from build123d import *

# Parameters (mm, degrees)
EXTRUDE_1_DEPTH = 100


with BuildPart() as part:
    # Model → 凸台-拉伸1 (new body)
    with BuildSketch(Plane.XY):
        with BuildLine():
            Line((1440.867570561, 579.107478259), (1452.807293918, 579.107478259))
            Line((1452.807293918, 579.107478259), (1457.807293918, 579.107478259))
            ThreePointArc((1457.807293918, 579.107478259), (1458.019425952, 579.019610294), (1458.107293918, 578.807478259))
            Line((1458.107293918, 578.807478259), (1458.107293918, 577.507478259))
            ThreePointArc((1458.107293918, 577.507478259), (1458.019425952, 577.295346225), (1457.807293918, 577.207478259))
            Line((1457.807293918, 577.207478259), (1408.407293918, 577.207478259))
            ThreePointArc((1408.407293918, 577.207478259), (1408.195161884, 577.295346225), (1408.107293918, 577.507478259))
            Line((1408.107293918, 577.507478259), (1408.107293918, 578.807478259))
            ThreePointArc((1408.107293918, 578.807478259), (1408.195161884, 579.019610294), (1408.407293918, 579.107478259))
            Line((1408.407293918, 579.107478259), (1425.347017276, 579.107478259))
            ThreePointArc((1425.347017276, 579.107478259), (1425.700570666, 579.253924869), (1425.847017276, 579.607478259))
            Line((1425.847017276, 579.607478259), (1425.847017276, 582.022074556))
            ThreePointArc((1425.847017276, 582.022074556), (1425.888989436, 582.222600109), (1426.007859266, 582.389459701))
            Line((1426.007859266, 582.389459701), (1427.136441813, 583.431330379))
            ThreePointArc((1427.136441813, 583.431330379), (1427.231524995, 583.680936543), (1427.089921929, 583.907415283))
            ThreePointArc((1427.089921929, 583.907415283), (1424.975565934, 585.575750276), (1423.307230942, 587.69010627))
            ThreePointArc((1423.307230942, 587.69010627), (1423.080752201, 587.831709337), (1422.831146038, 587.736626154))
            Line((1422.831146038, 587.736626154), (1421.789275359, 586.608043608))
            ThreePointArc((1421.789275359, 586.608043608), (1421.366754977, 586.450250809), (1420.989097485, 586.696821001))
            ThreePointArc((1420.989097485, 586.696821001), (1419.107293918, 593.707478259), (1420.989097485, 600.718135518))
            ThreePointArc((1420.989097485, 600.718135518), (1421.366754977, 600.96470571), (1421.789275359, 600.806912911))
            Line((1421.789275359, 600.806912911), (1422.831146038, 599.678330364))
            ThreePointArc((1422.831146038, 599.678330364), (1423.080752201, 599.583247182), (1423.307230942, 599.724850249))
            ThreePointArc((1423.307230942, 599.724850249), (1424.975565934, 601.839206243), (1427.089921929, 603.507541236))
            ThreePointArc((1427.089921929, 603.507541236), (1427.231524995, 603.734019976), (1427.136441813, 603.98362614))
            Line((1427.136441813, 603.98362614), (1426.007859266, 605.025496818))
            ThreePointArc((1426.007859266, 605.025496818), (1425.850066468, 605.448017201), (1426.096636659, 605.825674693))
            ThreePointArc((1426.096636659, 605.825674693), (1433.107293918, 607.707478259), (1440.117951177, 605.825674693))
            ThreePointArc((1440.117951177, 605.825674693), (1440.364521369, 605.448017201), (1440.20672857, 605.025496818))
            Line((1440.20672857, 605.025496818), (1439.078146023, 603.98362614))
            ThreePointArc((1439.078146023, 603.98362614), (1438.983062841, 603.734019976), (1439.124665907, 603.507541236))
            ThreePointArc((1439.124665907, 603.507541236), (1441.239021902, 601.839206243), (1442.907356895, 599.724850249))
            ThreePointArc((1442.907356895, 599.724850249), (1443.133835635, 599.583247182), (1443.383441798, 599.678330364))
            Line((1443.383441798, 599.678330364), (1444.425312477, 600.806912911))
            ThreePointArc((1444.425312477, 600.806912911), (1444.847832859, 600.96470571), (1445.225490352, 600.718135518))
            ThreePointArc((1445.225490352, 600.718135518), (1447.107293918, 593.707478259), (1445.225490352, 586.696821001))
            ThreePointArc((1445.225490352, 586.696821001), (1444.847832859, 586.450250809), (1444.425312477, 586.608043608))
            Line((1444.425312477, 586.608043608), (1443.383441798, 587.736626154))
            ThreePointArc((1443.383441798, 587.736626154), (1443.133835635, 587.831709337), (1442.907356895, 587.69010627))
            ThreePointArc((1442.907356895, 587.69010627), (1441.239021902, 585.575750276), (1439.124665907, 583.907415283))
            ThreePointArc((1439.124665907, 583.907415283), (1438.983062841, 583.680936543), (1439.078146023, 583.431330379))
            Line((1439.078146023, 583.431330379), (1440.20672857, 582.389459701))
            ThreePointArc((1440.20672857, 582.389459701), (1440.325598401, 582.222600109), (1440.367570561, 582.022074556))
            Line((1440.367570561, 582.022074556), (1440.367570561, 579.607478259))
            ThreePointArc((1440.367570561, 579.607478259), (1440.51401717, 579.253924869), (1440.867570561, 579.107478259))
        make_face()
        with BuildLine():
            Line((1421.166188442, 590.907478259), (1421.754066124, 590.907478259))
            ThreePointArc((1421.754066124, 590.907478259), (1421.914408846, 590.857021745), (1422.016963461, 590.723836915))
            Line((1422.016963461, 590.723836915), (1422.411999107, 589.64605289))
            ThreePointArc((1422.411999107, 589.64605289), (1422.514553722, 589.51286806), (1422.674896444, 589.462411545))
            Line((1422.674896444, 589.462411545), (1424.424991887, 589.462411545))
            ThreePointArc((1424.424991887, 589.462411545), (1424.58032957, 589.419063458), (1424.690776643, 589.30154624))
            ThreePointArc((1424.690776643, 589.30154624), (1426.389779497, 586.989963838), (1428.701361899, 585.290960984))
            ThreePointArc((1428.701361899, 585.290960984), (1428.818879117, 585.180513911), (1428.862227204, 585.025176228))
            Line((1428.862227204, 585.025176228), (1428.862227204, 583.275080785))
            ThreePointArc((1428.862227204, 583.275080785), (1428.912683718, 583.114738064), (1429.045868549, 583.012183448))
            Line((1429.045868549, 583.012183448), (1430.123652573, 582.617147802))
            ThreePointArc((1430.123652573, 582.617147802), (1430.256837404, 582.514593187), (1430.307293918, 582.354250466))
            Line((1430.307293918, 582.354250466), (1430.307293918, 581.766372783))
            ThreePointArc((1430.307293918, 581.766372783), (1430.374439218, 581.577220229), (1430.545818508, 581.472739042))
            ThreePointArc((1430.545818508, 581.472739042), (1433.107293918, 581.207478259), (1435.668769328, 581.472739042))
            ThreePointArc((1435.668769328, 581.472739042), (1435.840148618, 581.577220229), (1435.907293918, 581.766372783))
            Line((1435.907293918, 581.766372783), (1435.907293918, 582.354250466))
            ThreePointArc((1435.907293918, 582.354250466), (1435.957750433, 582.514593187), (1436.090935263, 582.617147802))
            Line((1436.090935263, 582.617147802), (1437.168719288, 583.012183448))
            ThreePointArc((1437.168719288, 583.012183448), (1437.301904118, 583.114738064), (1437.352360632, 583.275080785))
            Line((1437.352360632, 583.275080785), (1437.352360632, 585.025176228))
            ThreePointArc((1437.352360632, 585.025176228), (1437.39570872, 585.180513911), (1437.513225937, 585.290960984))
            ThreePointArc((1437.513225937, 585.290960984), (1439.824808339, 586.989963838), (1441.523811193, 589.30154624))
            ThreePointArc((1441.523811193, 589.30154624), (1441.634258267, 589.419063458), (1441.789595949, 589.462411545))
            Line((1441.789595949, 589.462411545), (1443.539691393, 589.462411545))
            ThreePointArc((1443.539691393, 589.462411545), (1443.700034114, 589.51286806), (1443.802588729, 589.64605289))
            Line((1443.802588729, 589.64605289), (1444.197624375, 590.723836915))
            ThreePointArc((1444.197624375, 590.723836915), (1444.300178991, 590.857021745), (1444.460521712, 590.907478259))
            Line((1444.460521712, 590.907478259), (1445.048399395, 590.907478259))
            ThreePointArc((1445.048399395, 590.907478259), (1445.237551948, 590.974623559), (1445.342033136, 591.14600285))
            ThreePointArc((1445.342033136, 591.14600285), (1445.607293918, 593.707478259), (1445.342033136, 596.268953669))
            ThreePointArc((1445.342033136, 596.268953669), (1445.237551948, 596.44033296), (1445.048399395, 596.507478259))
            Line((1445.048399395, 596.507478259), (1444.460521712, 596.507478259))
            ThreePointArc((1444.460521712, 596.507478259), (1444.300178991, 596.557934774), (1444.197624375, 596.691119604))
            Line((1444.197624375, 596.691119604), (1443.802588729, 597.768903629))
            ThreePointArc((1443.802588729, 597.768903629), (1443.700034114, 597.902088459), (1443.539691393, 597.952544974))
            Line((1443.539691393, 597.952544974), (1441.789595949, 597.952544974))
            ThreePointArc((1441.789595949, 597.952544974), (1441.634258267, 597.995893061), (1441.523811193, 598.113410278))
            ThreePointArc((1441.523811193, 598.113410278), (1440.851379085, 599.210127161), (1440.036940374, 600.205939616))
            Line((1440.036940374, 600.205939616), (1440.036940374, 600.637124715))
            Line((1440.036940374, 600.637124715), (1439.605755274, 600.637124715))
            ThreePointArc((1439.605755274, 600.637124715), (1438.609942819, 601.451563426), (1437.513225937, 602.123995535))
            ThreePointArc((1437.513225937, 602.123995535), (1437.39570872, 602.234442608), (1437.352360632, 602.389780291))
            Line((1437.352360632, 602.389780291), (1437.352360632, 604.139875734))
            ThreePointArc((1437.352360632, 604.139875734), (1437.301904118, 604.300218455), (1437.168719288, 604.402773071))
            Line((1437.168719288, 604.402773071), (1436.090935263, 604.797808717))
            ThreePointArc((1436.090935263, 604.797808717), (1435.957750433, 604.900363332), (1435.907293918, 605.060706053))
            Line((1435.907293918, 605.060706053), (1435.907293918, 605.648583736))
            ThreePointArc((1435.907293918, 605.648583736), (1435.840148618, 605.837736289), (1435.668769328, 605.942217477))
            ThreePointArc((1435.668769328, 605.942217477), (1433.107293918, 606.207478259), (1430.545818508, 605.942217477))
            ThreePointArc((1430.545818508, 605.942217477), (1430.374439218, 605.837736289), (1430.307293918, 605.648583736))
            Line((1430.307293918, 605.648583736), (1430.307293918, 605.060706053))
            ThreePointArc((1430.307293918, 605.060706053), (1430.256837404, 604.900363332), (1430.123652573, 604.797808717))
            Line((1430.123652573, 604.797808717), (1429.045868549, 604.402773071))
            ThreePointArc((1429.045868549, 604.402773071), (1428.912683718, 604.300218455), (1428.862227204, 604.139875734))
            Line((1428.862227204, 604.139875734), (1428.862227204, 602.389780291))
            ThreePointArc((1428.862227204, 602.389780291), (1428.818879117, 602.234442608), (1428.701361899, 602.123995535))
            ThreePointArc((1428.701361899, 602.123995535), (1426.389779497, 600.424992681), (1424.690776643, 598.113410278))
            ThreePointArc((1424.690776643, 598.113410278), (1424.58032957, 597.995893061), (1424.424991887, 597.952544974))
            Line((1424.424991887, 597.952544974), (1422.674896444, 597.952544974))
            ThreePointArc((1422.674896444, 597.952544974), (1422.514553722, 597.902088459), (1422.411999107, 597.768903629))
            Line((1422.411999107, 597.768903629), (1422.016963461, 596.691119604))
            ThreePointArc((1422.016963461, 596.691119604), (1421.914408846, 596.557934774), (1421.754066124, 596.507478259))
            Line((1421.754066124, 596.507478259), (1421.166188442, 596.507478259))
            ThreePointArc((1421.166188442, 596.507478259), (1420.977035888, 596.44033296), (1420.8725547, 596.268953669))
            ThreePointArc((1420.8725547, 596.268953669), (1420.607293918, 593.707478259), (1420.8725547, 591.14600285))
            ThreePointArc((1420.8725547, 591.14600285), (1420.977035888, 590.974623559), (1421.166188442, 590.907478259))
        make_face(mode=Mode.SUBTRACT)
    extrude(amount=EXTRUDE_1_DEPTH)


solid = part.part
Read the model definition and answer for the solid it produces. Units are mm, in the model's axes. A direction names the side the tool comes from. Coordinates: 2 decimals unless noted, no trailing zeros. Loops run counter-clockwise (first coordinate to the right, second up) from the corner with the lowest first, then second, coordinate; pieces in that order, holes last. Notation, with made-up numbers: (-7, 43.25) -> (21, 43.25) arc R30 cw to (21, 76.25) -> close; hole circle Ø6 at (44, -31). An arc over 180 degrees is marked (long way). Write item = value, one per line. Start each with the question number.
1) Given P1, Ø2, axis at y = 593, z = 23, coming from the -X side; P2, Ø13.5, axis at x = 1451, z = 30.5, coming from the +Y side; P3, Ø1.2, axis at y = 581.5, z = 59.5, coming from the -X side, each flat-ended and moving along its own axis, determine where each tip first touches the part or whether it passes through.
2) Find the intervals of material crossed by L1, parallel to Y at x = 1424, z = 13; L2, parallel to Y at x = 1442.5, z = 5.5; L3, parallel to X at y = 582, z = 46.5, in increasing order. Write a range as from..to.
3) For faces 4 (the face through (1425.847, 581, 49)), 5 (the face through (1445.607, 593.671, 49.3)), 6 (the face through (1440.368, 581, 49)), determine the directions among +Z, -Z, +X, -X, +Y, -Y from which every point of the face is accessible in a straight line to the end or side of a thin tool.
4) The part is cut by section A-A, the plane x = 1451.5. Determine the outline of the cut face in (y, z).
5) The mould has two halves that part along Y. Classify faces 1 (the face through (1433.004, 607.707, 49.3)), 2 (the face through (1439, 586, 0)), 3 (the face through (1449, 579.107, 49)): pulls with the +Y half, pulls with the -Y half, needs draft (parallel to the pull), parting line crosses it, or undercut.
Result:
q1.P1 = 1419.11
q1.P2 = 600.97
q1.P3 = 1425.85
q2.L1 = 577.21..579.11, 586.69..589.46, 597.95..600.73
q2.L2 = 577.21..579.11, 587.07..589.46, 597.95..600.34
q2.L3 = 1425.85..1430.31, 1435.91..1440.37
q3.face_4 = +Z, -Z, -X
q3.face_5 = +Z, -Z
q3.face_6 = +Z, -Z, +X
q4.outline = (577.21, 0) -> (579.11, 0) -> (579.11, 100) -> (577.21, 100) -> close
q5.face_1 = pulls with the +Y half
q5.face_2 = needs draft
q5.face_3 = undercut
